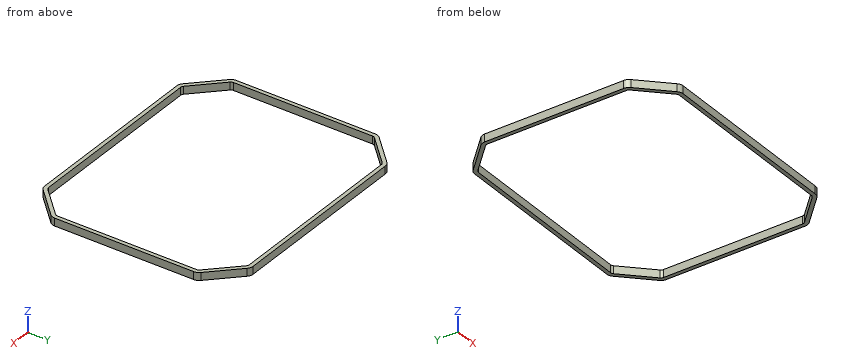
from build123d import *

# Parameters (mm, degrees)
BOSS_EXTRU_1_DEPTH = 2


with BuildPart() as part:
    # Esquisse1 → Boss.-Extru.1 (new body)
    with BuildSketch(Plane.XY):
        with BuildLine():
            Line((-24.001572875, -27), (24.001572875, -27))
            ThreePointArc((24.001572875, -27), (24.76693974, -26.847759065), (25.415786438, -26.414213562))
            Line((25.415786438, -26.414213562), (32.414213562, -19.415786438))
            ThreePointArc((32.414213562, -19.415786438), (32.847759065, -18.76693974), (33, -18.001572875))
            Line((33, -18.001572875), (33, 18.001572875))
            ThreePointArc((33, 18.001572875), (32.847759065, 18.76693974), (32.414213562, 19.415786438))
            Line((32.414213562, 19.415786438), (25.415786438, 26.414213562))
            ThreePointArc((25.415786438, 26.414213562), (24.76693974, 26.847759065), (24.001572875, 27))
            Line((24.001572875, 27), (-24.001572875, 27))
            ThreePointArc((-24.001572875, 27), (-24.76693974, 26.847759065), (-25.415786438, 26.414213562))
            Line((-25.415786438, 26.414213562), (-32.414213562, 19.415786438))
            ThreePointArc((-32.414213562, 19.415786438), (-32.847759065, 18.76693974), (-33, 18.001572875))
            Line((-33, 18.001572875), (-33, -18.001572875))
            ThreePointArc((-33, -18.001572875), (-32.847759065, -18.76693974), (-32.414213562, -19.415786438))
            Line((-32.414213562, -19.415786438), (-25.415786438, -26.414213562))
            ThreePointArc((-25.415786438, -26.414213562), (-24.76693974, -26.847759065), (-24.001572875, -27))
        make_face()
        with BuildLine():
            Line((24.001572875, 26), (-24.001572875, 26))
            ThreePointArc((-24.001572875, 26), (-24.384256308, 25.923879533), (-24.708679656, 25.707106781))
            Line((-24.708679656, 25.707106781), (-31.707106781, 18.708679656))
            ThreePointArc((-31.707106781, 18.708679656), (-31.923879533, 18.384256308), (-32, 18.001572875))
            Line((-32, 18.001572875), (-32, -18.001572875))
            ThreePointArc((-32, -18.001572875), (-31.923879533, -18.384256308), (-31.707106781, -18.708679656))
            Line((-31.707106781, -18.708679656), (-24.708679656, -25.707106781))
            ThreePointArc((-24.708679656, -25.707106781), (-24.384256308, -25.923879533), (-24.001572875, -26))
            Line((-24.001572875, -26), (24.001572875, -26))
            ThreePointArc((24.001572875, -26), (24.384256308, -25.923879533), (24.708679656, -25.707106781))
            Line((24.708679656, -25.707106781), (31.707106781, -18.708679656))
            ThreePointArc((31.707106781, -18.708679656), (31.923879533, -18.384256308), (32, -18.001572875))
            Line((32, -18.001572875), (32, 18.001572875))
            ThreePointArc((32, 18.001572875), (31.923879533, 18.384256308), (31.707106781, 18.708679656))
            Line((31.707106781, 18.708679656), (24.708679656, 25.707106781))
            ThreePointArc((24.708679656, 25.707106781), (24.384256308, 25.923879533), (24.001572875, 26))
        make_face(mode=Mode.SUBTRACT)
    extrude(amount=BOSS_EXTRU_1_DEPTH)


solid = part.part
CAD build for the part. Positions are in the model's coordinates, mm. Coordinates: 2 decimals unless noted, no trailing zeros. Write each loop counter-clockwise with the first axis right and the second up, starting at its lowest first coordinate (ties: lowest second). Pieces come first, ordered by that corner, then holes. Notation, with made-up numbers: (15.5, 47.25) - (32.5, 47.25) arc R11 cw to (32.5, 62.25) - close; hole circle Ø11 at (53.5, 18.5). An arc over 180 degrees is marked (long way). Use a Markdown table: item, result. Add a question column.
Item 1: Drill centre lines: L1, parallel to Y at x = 20, z = 1.7; L2, parallel to X at y = -6, z = 1.85; L3, parallel to X at y = -19.5, z = 0.7. Where is each one in solid material? Low to high. Write a range as from..to.
Item 2: Band-saw the part on A-A, the plane x = -5. Give the cut face in (y, z).
Item 3: Band-saw the part on C-C, the plane y = 14.5. Give the cut face in (x, z).
Numbers:
| question | item | result |
|---|---|---|
| 1 | L1 | -27..-26, 26..27 |
| 1 | L2 | -33..-32, 32..33 |
| 1 | L3 | -32.33..-30.92, 30.92..32.33 |
| 2 | outline | (-27, 0) - (-26, 0) - (-26, 2) - (-27, 2) - close; (26, 0) - (27, 0) - (27, 2) - (26, 2) - close |
| 3 | outline | (-33, 0) - (-32, 0) - (-32, 2) - (-33, 2) - close; (32, 0) - (33, 0) - (33, 2) - (32, 2) - close |
